Build history of the part. All positions in model axes, mm. Face numbers are marked on the shaded views. A direction names the side the tool comes from. Round coordinates to 2 decimals unless told otherwise and drop trailing zeros. Write each loop counter-clockwise with the first axis right and the second up, starting at its lowest first coordinate (ties: lowest second). Pieces come first, ordered by that corner, then holes. Notation, with made-up numbers: M 15.5,-40 L 73.5,-40 A18 cw 73.5,-5 Z; hole C 11,-20.75 d11. An arc over 180 degrees is marked long. One line per item, written item: value. Start each with the question number.
```python
from build123d import *

# Parameters (mm, degrees)
F2_DEPTH = 10
F1_W     = 26
F1_H     = 12
F3_DEPTH = 5
F4_D     = 3


with BuildPart() as f2:
    # F1 (on Top) → F2 (new body)
    with BuildSketch(Plane.XY):
        Polygon((20.9, 30.9), (20.9, 16.5), (17.9, 16.5), (17.9, 13.2), (19.4, 11.7), (20.9, 11.7), (20.9, 4.9), (14.1, 4.9), (14.1, 6.4), (12.6, 7.9), (9.3, 7.9), (9.3, 4.9), (-5.1, 4.9), (-5.1, -0.1), (20.9, -0.1), (25.9, 4.9), (25.9, 30.9), align=None)
    extrude(amount=F2_DEPTH)

    # F1 (on Top) → F3 (join)
    with BuildSketch(Plane.XY):
        with Locations((7.9, -6.1)):
            Rectangle(F1_W, F1_H)
    extrude(amount=F3_DEPTH)

    # F4 (through all)
    with Locations(Plane(origin=(0, 0, 0), x_dir=(1, 0, 0), z_dir=(0, 0, -1))):
        with Locations((7.8999996185, 8.1)):
            Hole(F4_D / 2)


solid = f2.part
```
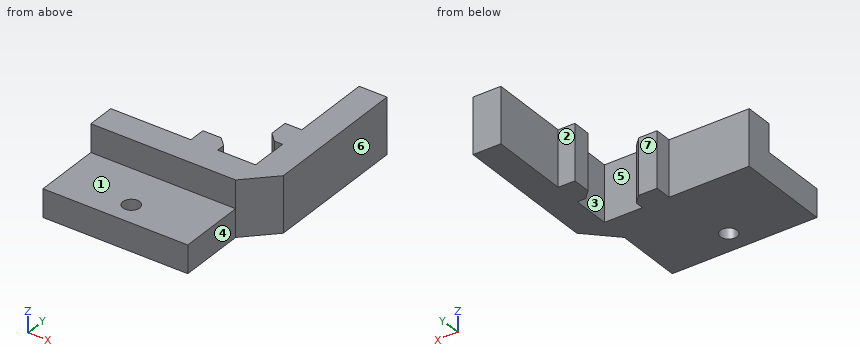
Item 1: Drop flat-ended pins along their axis: pin 1 (6 mm diameter, centred on x = 6, y = -4.5, fed in from +Z); pin 2 (3.5 mm diameter, centred on y = 9.5, z = 5, fed in from -X); pin 3 (4 mm diameter, centred on y = -3.5, z = 8.5, fed in from -X); pin 4 (3.5 mm diameter, centred on x = 18.5, z = 4.5, fed in from +Y). Give the stop position or say it passes through.
Item 2: Two-plate mould, pull along X, no slides. Class the marked faces 5, 6 and 7: pulls with the +X half, pulls with the -X half, needs draft (parallel to the pull), parting line crosses it, or undercut.
Item 3: Cut at C-C, the plane z = 7.5. Write the cut outline in (x, y).
Item 4: Cut at B-B, the plane y = -8.1. Write the cut outline in (x, z), plus the area to 3 significant figures.
Item 5: Drill centre lines: line 1 (Y direction, x = 18.5, z = 6); line 2 (Y direction, x = 7.9, z = 1.7); line 3 (X direction, y = -8.1, z = 2.55). Where is each one in solid material? Low to high.
Item 6: Cut at D-D, the plane z = 1. Write the cut outline in (x, y).
Item 7: Cut at A-A, the plane x = 7.9. Write the cut outline in (y, z).
Item 8: Which spindle directions (+Z, -Z, +X, -X, +Y, -Y) get a long thin tool onto all of the face, cutting with end or side? Do the marked faces 1, 2, 3 and 4. Say none if no direction does.
Computed values:
1. pin 1: stops at z = 5
1. pin 2: stops at x = 9.3
1. pin 3: passes through
1. pin 4: stops at y = 16.5
2. face 5: undercut
2. face 6: pulls with the +X half
2. face 7: needs draft
3. outline: M -5.1,-0.1 L 20.9,-0.1 L 25.9,4.9 L 25.9,30.9 L 20.9,30.9 L 20.9,16.5 L 17.9,16.5 L 17.9,13.2 L 19.4,11.7 L 20.9,11.7 L 20.9,4.9 L 14.1,4.9 L 14.1,6.4 L 12.6,7.9 L 9.3,7.9 L 9.3,4.9 L -5.1,4.9 Z
4. outline: M -5.1,0 L 6.4,0 L 6.4,5 L -5.1,5 Z; M 9.4,0 L 20.9,0 L 20.9,5 L 9.4,5 Z
4. area: 115 mm2
5. line 1: y = -0.1 to 4.9, 12.6 to 16.5
5. line 2: y = -12.1 to -9.6, -6.6 to 4.9
5. line 3: x = -5.1 to 6.4, 9.4 to 20.9
6. outline: M -5.1,-12.1 L 20.9,-12.1 L 20.9,-0.1 L 25.9,4.9 L 25.9,30.9 L 20.9,30.9 L 20.9,16.5 L 17.9,16.5 L 17.9,13.2 L 19.4,11.7 L 20.9,11.7 L 20.9,4.9 L 14.1,4.9 L 14.1,6.4 L 12.6,7.9 L 9.3,7.9 L 9.3,4.9 L -5.1,4.9 Z; hole C 7.9,-8.1 d3
7. outline: M -12.1,0 L -9.6,0 L -9.6,5 L -12.1,5 Z; M -6.6,0 L 4.9,0 L 4.9,10 L -0.1,10 L -0.1,5 L -6.6,5 Z
8. face 1: +Z, +X, -X, -Y
8. face 2: +Z, -Z, -X, +Y
8. face 3: +Z, -Z
8. face 4: +Z, -Z, +X, -Y
